Input: dimensioned drawing with shaded views. Units: mm. Origin: part minimum x, y, z. Give positions to 0.01 mm unless a question says otherwise; leave off trailing zeros. Write each loop counter-clockwise with the first axis right and the second up, starting at its lowest first coordinate (ties: lowest second). Pieces come first, ordered by that corner, then holes.
Q1. Section C-C (y = 1.8). Return the cut outline in (x, z) (1 decimal).
Q2. Section B-B (x = 30). Return the cut outline in (y, z), plus the area to 3 significant figures.
Q3. Section A-A (z = 10). Return the cut outline in (x, y).
Q4. Pin query (flat end, axial travel): pin 1 Ø1.5 at (y, z) = (0.5, 29.5) entering from +X; pin 2 Ø1 at (y, z) = (1.5, 54) entering from -X; pin 3 Ø5 at (x, z) = (10, 10) entering from +Y. Return the tip coordinate at first contact, or that it passes through.
Q5. Section D-D (z = 65). Return the cut outline in (x, y).
Q6. Line query: line 1 (Z direction, x = 50, y = 0.25); line 2 (X direction, y = 0.8, z = 10); line 3 (X direction, y = 0.6, z = 65). Output: solid intervals per line, ascending.
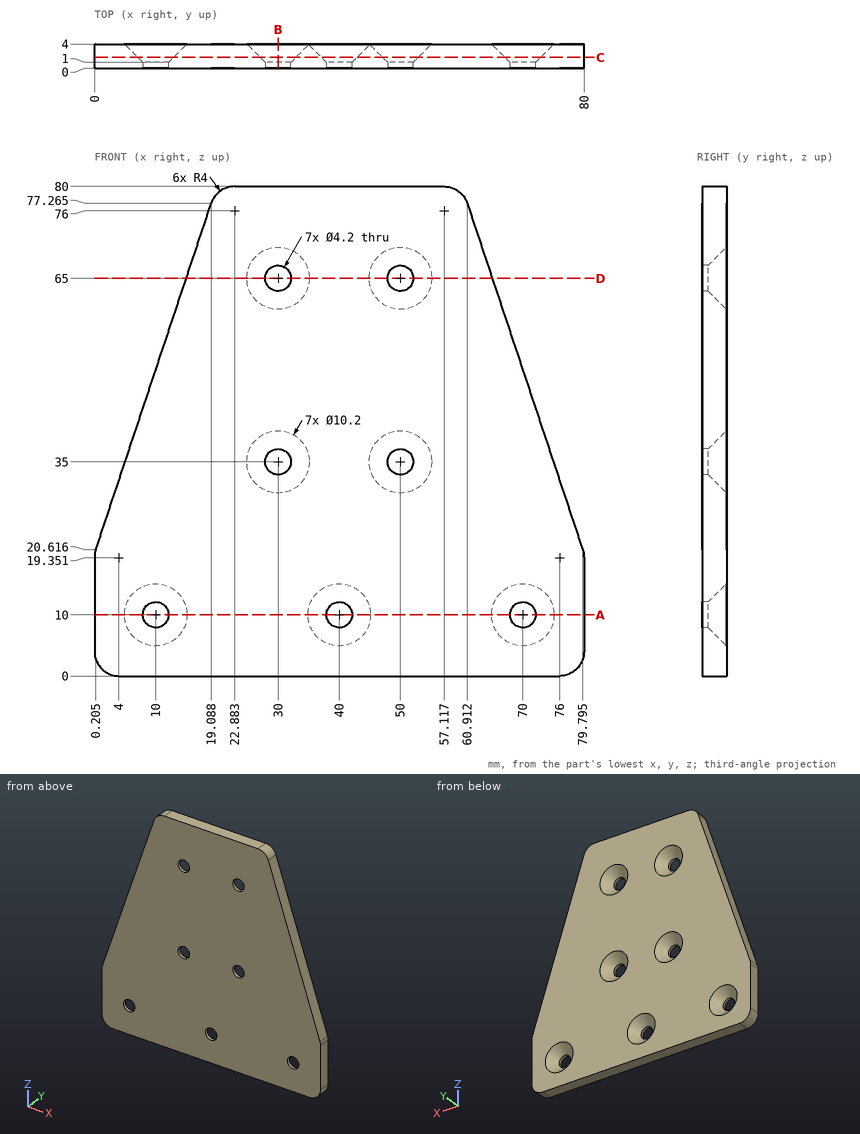
Computed:
1. outline: (0, 4) arc R4 ccw to (4, 0) - (76, 0) arc R4 ccw to (80, 4) - (80, 19.4) arc R4 ccw to (79.8, 20.6) - (60.9, 77.3) arc R4 ccw to (57.1, 80) - (22.9, 80) arc R4 ccw to (19.1, 77.3) - (0.2, 20.6) arc R4 ccw to (0, 19.4) - close; hole circle Ø5.8 at (10, 10); hole circle Ø5.8 at (30, 35); hole circle Ø5.8 at (30, 65); hole circle Ø5.8 at (40, 10); hole circle Ø5.8 at (50, 35); hole circle Ø5.8 at (50, 65); hole circle Ø5.8 at (70, 10)
2. outline: (0, 0) - (4, 0) - (4, 29.9) - (1, 32.9) - (0, 32.9) - close; (0, 37.1) - (1, 37.1) - (4, 40.1) - (4, 59.9) - (1, 62.9) - (0, 62.9) - close; (0, 67.1) - (1, 67.1) - (4, 70.1) - (4, 80) - (0, 80) - close
2. area: 268 mm2
3. outline: (0, 0) - (7.9, 0) - (7.9, 1) - (4.9, 4) - (0, 4) - close; (12.1, 0) - (37.9, 0) - (37.9, 1) - (34.9, 4) - (15.1, 4) - (12.1, 1) - close; (42.1, 0) - (67.9, 0) - (67.9, 1) - (64.9, 4) - (45.1, 4) - (42.1, 1) - close; (72.1, 0) - (80, 0) - (80, 4) - (75.1, 4) - (72.1, 1) - close
4. pin 1: stops at x = 77.08
4. pin 2: stops at x = 11.17
4. pin 3: stops at y = 1.4
5. outline: (15, 0) - (27.9, 0) - (27.9, 1) - (24.9, 4) - (15, 4) - close; (32.1, 0) - (47.9, 0) - (47.9, 1) - (44.9, 4) - (35.1, 4) - (32.1, 1) - close; (52.1, 0) - (65, 0) - (65, 4) - (55.1, 4) - (52.1, 1) - close
6. line 1: z = 0 to 32.9, 37.1 to 62.9, 67.1 to 80
6. line 2: x = 0 to 7.9, 12.1 to 37.9, 42.1 to 67.9, 72.1 to 80
6. line 3: x = 15 to 27.9, 32.1 to 47.9, 52.1 to 65
